```python
from build123d import *

# Parameters (mm, degrees)
SKETCH1_W           = 45
SKETCH1_H           = 7
BOSS_EXTRUDE1_DEPTH = 5
SKETCH2_W           = 37
SKETCH2_H           = 7
BOSS_EXTRUDE2_DEPTH = 5
FILLET1_R           = 5
SKETCH3_W           = 22
SKETCH3_H           = 10
BOSS_EXTRUDE3_DEPTH = 5
FILLET2_R           = 5
SKETCH4_W           = 12.1
SKETCH4_H           = 5.1
CUT_EXTRUDE1_DEPTH  = 2.1


with BuildPart() as part:
    # Sketch1 → Boss-Extrude1 (new body)
    with BuildSketch(Plane.XY):
        Rectangle(SKETCH1_W, SKETCH1_H)
    extrude(amount=BOSS_EXTRUDE1_DEPTH)

    # Sketch2 → Boss-Extrude2 (add)
    with BuildSketch(Plane.ZY.offset(22.5)):
        with Locations((-13.5, 0)):
            Rectangle(SKETCH2_W, SKETCH2_H)
    extrude(amount=BOSS_EXTRUDE2_DEPTH)

    # Fillet1
    fillet1_edges = [part.edges().sort_by_distance(p)[0] for p in [
        (-27.5, 0, 5),
    ]]
    fillet(fillet1_edges, radius=FILLET1_R)

    # Sketch3 → Boss-Extrude3 (add)
    with BuildSketch(Plane(origin=(22.5, 0, 0), x_dir=(0, 0, -1), z_dir=(1, 0, 0))):
        with Locations((-11, 1.5)):
            Rectangle(SKETCH3_W, SKETCH3_H)
    extrude(amount=BOSS_EXTRUDE3_DEPTH)

    # Fillet2
    fillet2_edges = [part.edges().sort_by_distance(p)[0] for p in [
        (27.5, 1.5, 0),
    ]]
    fillet(fillet2_edges, radius=FILLET2_R)

    # Sketch4 → Cut-Extrude1 (cut)
    with BuildSketch(Plane(origin=(-22.5, 0, 0), x_dir=(0, 0, -1), z_dir=(1, 0, 0))):
        with Locations((24.95, 0.05)):
            Rectangle(SKETCH4_W, SKETCH4_H)
    extrude(amount=-CUT_EXTRUDE1_DEPTH, mode=Mode.SUBTRACT)


solid = part.part
```
Build history of the part. All positions in model axes, mm. A direction names the side the tool comes from. Give positions to 0.01 mm unless a question says otherwise; leave off trailing zeros. Loops run counter-clockwise (first coordinate to the right, second up) from the corner with the lowest first, then second, coordinate; pieces in that order, holes last.
1) Band-saw the part on D-D on z = 3. List the corners of the cut face in (x, y).
Values follow:
outline: (-26.5, -3.5) - (27.08, -3.5) - (27.08, 6.5) - (22.5, 6.5) - (22.5, 3.5) - (-26.5, 3.5) - close
2) Drop flat-ended pins along their axis: P1, Ø4, axis at y = 0.5, z = -27.5, coming from the +X side; P2, Ø1, axis at y = 2, z = 12, coming from the -X side; P3, Ø3, axis at x = -18, y = 1.5, coming from the -Z side. Give the stop position or say it passes through.
Values follow:
P1: stops at x = -24.6
P2: stops at x = 22.5
P3: stops at z = 0
3) 3-axis set-ups, long thin cutter, end or side, ignore diameter. For faces 1 (the face through (-24, 0, -18.9)), 2 (the face through (0, 0, 0)), 3 (the face through (0, 0, 5)): which of +Z, -Z, +X, -X, +Y, -Y reach the whole face in a straight line?
Values follow:
face 1: +X
face 2: -Z, +X, +Y, -Y
face 3: +Z, -X, +Y, -Y
4) Probe line 1 along X through (y, z) = (-0.75, -9); line 2 along Z through (x, y) = (-1, 1.75); line 3 along X through (y, z) = (-3, 18.5). List the from-to ranges inside material, lowest first.
Values follow:
line 1: x = -27.5 to -22.5
line 2: z = 0 to 5
line 3: x = 22.5 to 27.5
5) Two-plate mould, pull along Y, no slides. Class faces 4 (the face through (-12, 3.5, 1)), 5 (the face through (-25, 0, -32)), 6 (the face through (-24, -2.5, -25)): released by +Y, released by -Y, zero draft, split by the parting line, or undercut.
Values follow:
face 4: released by +Y
face 5: zero draft
face 6: undercut
6) Band-saw the part on A-A on y = 1. List the corners of the cut face in (x, z).
Values follow:
outline: (-27.5, -32) - (-22.5, -32) - (-22.5, -31) - (-24.6, -31) - (-24.6, -18.9) - (-22.5, -18.9) - (-22.5, 0) - (22.5, 0) arc R5 ccw to (27.5, 5) - (27.5, 22) - (22.5, 22) - (22.5, 5) - (-22.5, 5) arc R5 ccw to (-27.5, 0) - close
7) Band-saw the part on B-B on z = -17. List the corners of the cut face in (x, y).
Values follow:
outline: (-27.5, -3.5) - (-22.5, -3.5) - (-22.5, 3.5) - (-27.5, 3.5) - close
8) Band-saw the part on C-C on x = -3. List the corners of the cut face in (y, z).
Values follow:
outline: (-3.5, 0) - (3.5, 0) - (3.5, 5) - (-3.5, 5) - close
